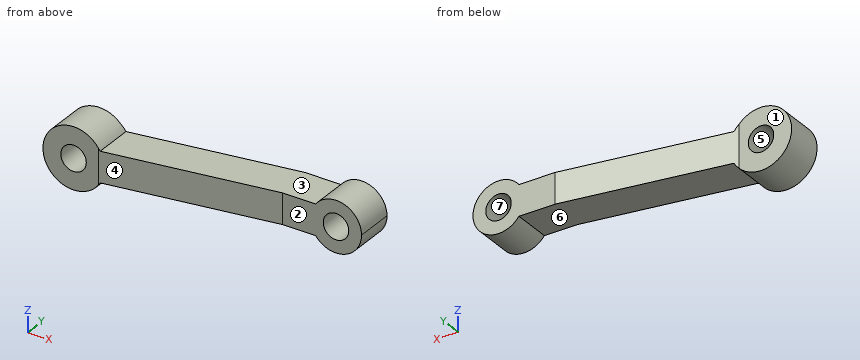
```python
from build123d import *

# Parameters (mm, degrees)
F0_R     = 7.9375
F1_DEPTH = 23.368
F3_DEPTH = 25.4


with BuildPart() as f1:
    # F0 (on Front) → F1 (new body, symmetric)
    with BuildSketch(Plane.XZ):
        with BuildLine():
            ThreePointArc((16.497784, -9.525), (18.400887, -4.930503), (19.05, 0))
            ThreePointArc((19.05, 0), (18.400887, 4.930503), (16.497784, 9.525))
            ThreePointArc((16.497784, 9.525), (-19.05, 0), (16.497784, -9.525))
        make_face()
        Circle(F0_R, mode=Mode.SUBTRACT)
        with BuildLine():
            ThreePointArc((16.497784, 9.525), (18.400887, 4.930503), (19.05, 0))
            ThreePointArc((19.05, 0), (18.400887, -4.930503), (16.497784, -9.525))
            Line((16.497784, -9.525), (139.7, -9.525))
            ThreePointArc((139.7, -9.525), (136.525, 0), (139.7, 9.525))
            Line((139.7, 9.525), (16.497784, 9.525))
        make_face()
        with BuildLine():
            ThreePointArc((168.275, 0), (157.420116, 15.060347), (139.7, 9.525))
            ThreePointArc((139.7, 9.525), (136.525, 0), (139.7, -9.525))
            ThreePointArc((139.7, -9.525), (157.420116, -15.060347), (168.275, 0))
        make_face()
        with Locations((152.4, 0)):
            Circle(F0_R, mode=Mode.SUBTRACT)
    extrude(amount=F1_DEPTH, both=True)

    # F2 (on Top) → F3 (intersect, symmetric)
    with BuildSketch(Plane.XY):
        Polygon((-19.05, -23.368), (-19.05, -23.392219), (15.476332, -23.392219), (119.003983, -6.732617), (168.275, -6.732617), (168.275, 17.229946), (117.088285, 17.229946), (13.560635, 0.570344), (-19.05, 0.570344), (-19.05, -18.542036), align=None)
    extrude(amount=F3_DEPTH, both=True, mode=Mode.INTERSECT)


solid = f1.part
```
The model under review builds one solid part; all positions refer to its coordinate system, in mm. Face numbers are marked on the shaded views. A direction names the side the tool comes from. Coordinates: 2 decimals unless noted, no trailing zeros. Write each loop counter-clockwise with the first axis right and the second up, starting at its lowest first coordinate (ties: lowest second). Pieces come first, ordered by that corner, then holes.
1) We need section A-A on x = 0. State the section outline as (y, z) points.
2) We need section C-C on z = 2. State the section outline as (x, y) points, then the cut area to 3 significant figures.
3) The part is to be moulded in two halves that separate along Z. For the marked faces 4, 5, 6 and 7, say which applies: pulls with the +Z half, pulls with the -Z half, needs draft (parallel to the pull), parting line crosses it, or undercut.
4) Machinability: for the marked faces 1, 2 and 3, which of the approach directions +Z, -Z, +X, -X, +Y, -Y give a long, thin tool a straight path to every point of the face, cutting with its end or side? Answer none if there is none.
5) To check wall thickness, follow probe 1 along Z at (x, y) = (0, -17.5); probe 2 along Z at (x, y) = (152.4, 12.5) (1 decimal); probe 3 along Z at (x, y) = (48.5, -6) (3 decimals). State the ranges of each line that lie inside material, in increasing order.
6) Clearance check with flat-ended pins moving along their axes: pin 1 Ø8 at (x, z) = (88.5, -2.5) entering from +Y; pin 2 Ø3 at (x, y) = (3, -9) entering from -Z; pin 3 Ø20.5 at (x, z) = (152.4, 0) entering from -Y; pin 4 Ø1 at (x, y) = (133, -7.5) entering from +Z. State where each tip first meets the part, or that it passes through.
7) We need section D-D on x = 152.4. State the section outline as (y, z) points (1 decimal).
Answer list:
1. outline: (-23.37, -19.05) - (0.57, -19.05) - (0.57, -7.94) - (-23.37, -7.94) - close; (-23.37, 7.94) - (0.57, 7.94) - (0.57, 19.05) - (-23.37, 19.05) - close
2. outline: (-18.94, -23.37) - (-7.68, -23.37) - (-7.68, 0.57) - (-18.94, 0.57) - close; (7.68, -23.37) - (15.63, -23.37) - (119, -6.73) - (144.72, -6.73) - (144.72, 17.23) - (117.09, 17.23) - (13.56, 0.57) - (7.68, 0.57) - close; (160.08, -6.73) - (168.15, -6.73) - (168.15, 17.23) - (160.08, 17.23) - close
2. area: 3,780 mm2
3. face 4: needs draft
3. face 5: undercut
3. face 6: pulls with the -Z half
3. face 7: undercut
4. face 1: +Z, -Z, -X, +Y
4. face 2: +Z, -Z, +X, -Y
4. face 3: +Z, +Y, -Y
5. probe 1: z = -19.05 to -7.94, 7.94 to 19.05
5. probe 2: z = -15.9 to -7.9, 7.9 to 15.9
5. probe 3: z = -9.525 to 9.525
6. pin 1: stops at y = 13.27
6. pin 2: stops at z = -18.99
6. pin 3: stops at y = -6.73
6. pin 4: passes through
7. outline: (-6.7, -15.9) - (17.2, -15.9) - (17.2, -7.9) - (-6.7, -7.9) - close; (-6.7, 7.9) - (17.2, 7.9) - (17.2, 15.9) - (-6.7, 15.9) - close
